Can you work these out from the model? Positions are in its coordinate system, mm. A direction names the side the tool comes from. Round coordinates to 2 decimals unless told otherwise and drop trailing zeros. Loops run counter-clockwise (first coordinate to the right, second up) from the corner with the lowest first, then second, coordinate; pieces in that order, holes last. Notation, with made-up numbers: M 35.25,34.5 L 86.25,34.5 A26 ccw 86.25,58.5 Z; hole C 47,-29 d3. An arc over 180 degrees is marked long. Answer as CSV lines item,"result".
from build123d import *

# Parameters (mm, degrees)
F0_R      = 63.5
F1_DEPTH  = 6.35
F2_R      = 1.5875
F3_DEPTH  = 6.351
F6_R      = 2.778125
F7_DEPTH  = 44.45
F8_COUNT  = 8
F10_DEPTH = 1.5875
F4_R      = 63.5
F4_R_2    = 1.5875
F11_DEPTH = 1.5875
F12_DEPTH = 2.38125
F13_DEPTH = 2.38125


with BuildPart() as f1:
    # F0 (on Front) → F1 (new body)
    with BuildSketch(Plane.XZ):
        Circle(F0_R)
    extrude(amount=F1_DEPTH)

    # F2 (on face) → F3 (cut, through all)
    with BuildSketch(Plane.XZ.offset(6.35)):
        Circle(F2_R)
    extrude(amount=-F3_DEPTH, mode=Mode.SUBTRACT)


with BuildPart() as f7:
    # F6 (on line) → F7 (new body)
    with BuildSketch(Plane.YZ.offset(63.5)):
        with Locations((-3.175, 0)):
            Circle(F6_R)
    extrude(amount=-F7_DEPTH)


with BuildPart() as f8_1:
    # F8: instance of F7
    add(f7.part.rotate(Axis((0, -6.35, 0), (0, -1, 0)), 1 * 360 / F8_COUNT))


with BuildPart() as f8_2:
    # F8: instance of F7
    add(f7.part.rotate(Axis((0, -6.35, 0), (0, -1, 0)), 2 * 360 / F8_COUNT))


with BuildPart() as f8_3:
    # F8: instance of F7
    add(f7.part.rotate(Axis((0, -6.35, 0), (0, -1, 0)), 3 * 360 / F8_COUNT))


with BuildPart() as f8_4:
    # F8: instance of F7
    add(f7.part.rotate(Axis((0, -6.35, 0), (0, -1, 0)), 4 * 360 / F8_COUNT))


with BuildPart() as f8_5:
    # F8: instance of F7
    add(f7.part.rotate(Axis((0, -6.35, 0), (0, -1, 0)), 5 * 360 / F8_COUNT))


with BuildPart() as f8_6:
    # F8: instance of F7
    add(f7.part.rotate(Axis((0, -6.35, 0), (0, -1, 0)), 6 * 360 / F8_COUNT))


with BuildPart() as f8_7:
    # F8: instance of F7
    add(f7.part.rotate(Axis((0, -6.35, 0), (0, -1, 0)), 7 * 360 / F8_COUNT))


with BuildPart() as f1_1:
    add(f1.part)

    # F9: cut F8_1, F7, F8_7, F8_2, F8_3, F8_4, F8_5, F8_6
    add(f8_1.part, mode=Mode.SUBTRACT)
    add(f7.part, mode=Mode.SUBTRACT)
    add(f8_7.part, mode=Mode.SUBTRACT)
    add(f8_2.part, mode=Mode.SUBTRACT)
    add(f8_3.part, mode=Mode.SUBTRACT)
    add(f8_4.part, mode=Mode.SUBTRACT)
    add(f8_5.part, mode=Mode.SUBTRACT)
    add(f8_6.part, mode=Mode.SUBTRACT)

    # F10 (add): a face of the model
    f10_faces = [f1_1.faces().sort_by_distance(p)[0] for p in [
        (-61.7039487758, -6.35, 0),
    ]]
    extrude(f10_faces, amount=F10_DEPTH)

    # F4 (on face) → F11 (join)
    with BuildSketch(Plane(origin=(0, 0, 0), x_dir=(-1, 0, 0), z_dir=(0, 1, 0))):
        Circle(F4_R)
        Circle(F4_R_2, mode=Mode.SUBTRACT)
    extrude(amount=F11_DEPTH)

    # F12 (add): a face of the model
    f12_faces = [f1_1.faces().sort_by_distance(p)[0] for p in [
        (-61.7039487758, -7.9375, 0),
    ]]
    extrude(f12_faces, amount=F12_DEPTH)

    # F13 (add): a face of the model
    f13_faces = [f1_1.faces().sort_by_distance(p)[0] for p in [
        (61.7039487758, 1.5875, 0),
    ]]
    extrude(f13_faces, amount=F13_DEPTH)


solid = f1_1.part
Item 1: If we section it at D-D on z = -26: State how many separate pieces and enclosed holes the cut face has, then the cut area to 3 significant figures.
Output:
separate pieces,"1"
enclosed holes,"3"
area,"1,560 mm2"
Item 2: Will these pins go through, and if not, where does the flat tip stop? pin 1 (1 mm diameter, centred on y = -2, z = 36.5, fed in from -X); pin 2 (6 mm diameter, centred on y = -6, z = 10, fed in from -X); pin 3 (4.5 mm diameter, centred on x = 0, y = -3.175, fed in from +Z).
Output:
pin 1,"stops at x = -52.31"
pin 2,"stops at x = -63.11"
pin 3,"stops at z = 19.05"
Item 3: If I drill on line 1 along X through (y, z) = (-1.75, 0); line 2 along X through (y, z) = (-1.25, -31); line 3 along X through (y, z) = (-2, -40), over which ranges is the centre line in solid material (lowest first)? Write a range as from..to.
Output:
line 1,"x = -19.05..-1.59, 1.59..19.05"
line 2,"x = -55.42..-33.83, -28.17..-2, 2..28.17, 33.83..55.42"
line 3,"x = -49.32..-43.56, -36.44..-2.52, 2.52..36.44, 43.56..49.32"
Item 4: If we section it at B-B on z = 0: Write out the boundary of the cut face in (x, y), then the cut area to 3 significant figures.
Output:
outline,"M -63.5,-10.32 L -1.59,-10.32 L -1.59,3.97 L -63.5,3.97 L -63.5,-0.4 L -19.05,-0.4 L -19.05,-5.95 L -63.5,-5.95 Z; M 1.59,-10.32 L 63.5,-10.32 L 63.5,-5.95 L 19.05,-5.95 L 19.05,-0.4 L 63.5,-0.4 L 63.5,3.97 L 1.59,3.97 Z"
area,"1,280 mm2"
Item 5: If we section it at A-A on x = 0: Write out the boundary of the cut face in (y, z), then the cut area to 3 significant figures.
Output:
outline,"M -10.32,-63.5 L -5.95,-63.5 L -5.95,-19.05 L -0.4,-19.05 L -0.4,-63.5 L 3.97,-63.5 L 3.97,-1.59 L -10.32,-1.59 Z; M -10.32,1.59 L 3.97,1.59 L 3.97,63.5 L -0.4,63.5 L -0.4,19.05 L -5.95,19.05 L -5.95,63.5 L -10.32,63.5 Z"
area,"1,280 mm2"
Item 6: We'd pull the mould along X, two halves only. Please class faces 1 (the face through (-19.05, -3, 0)), 2 (the face through (-1.064, -0.609, -41.586)), 3 (the face through (-13, 3.969, 1)): released by +X, released by -X, zero draft, split by the parting line, or undercut.
Output:
face 1,"released by -X"
face 2,"undercut"
face 3,"zero draft"
Item 7: On a 3-axis mill with a long thin cutter (end or side, diameter ignored), from which of +Z, -Z, +X, -X, +Y, -Y can I reach the whole of each face in a straight line? I mean faces 4 (the face through (0, -3, -19.05)), 5 (the face through (41.586, -0.525, 0.834)), 6 (the face through (-13.5, -3.21, 13.44)). Say none if no direction works.
Output:
face 4,"-Z"
face 5,"+X"
face 6,"none"
Item 8: If we section it at C-C on x = -48.5: Write out the boundary of the cut face in (y, z) (3 decimals), then the cut area to 3 significant figures.
Output:
outline,"M -10.319,-40.988 L 3.969,-40.988 L 3.969,40.988 L -10.319,40.988 Z; hole C -3.175,0 d5.556"
area,"1,150 mm2"
